```python
from build123d import *

# Parameters (mm, degrees)
BOSS_EXTRUDE1_DEPTH = 30
SKETCH2_R           = 7
SKETCH2_R_2         = 1.5
CUT_EXTRUDE1_DEPTH  = 55
SKETCH3_R           = 3
CUT_EXTRUDE2_DEPTH  = 55
SKETCH4_W           = 8
SKETCH4_H           = 40
BOSS_EXTRUDE2_DEPTH = 60
SKETCH5_R           = 2.5
CUT_EXTRUDE3_DEPTH  = 10
SKETCH6_W           = 8
SKETCH6_H           = 7.5
CUT_EXTRUDE4_DEPTH  = 94.808315196


with BuildPart() as part:
    # Sketch1 → Boss-Extrude1 (new, symmetric)
    with BuildSketch(Plane(origin=(0, 0, 0), x_dir=(0, 0, -1), z_dir=(1, 0, 0))):
        Polygon((0, 20), (0, 0), (-52, 0), (-52, -8), (8, -8), (8, 20), align=None)
    extrude(amount=BOSS_EXTRUDE1_DEPTH, both=True)

    # Sketch2 → Cut-Extrude1 (cut)
    with BuildSketch(Plane(origin=(0, 0, 0), x_dir=(1, 0, 0), z_dir=(0, 1, 0))):
        with Locations(Location((0, -37, 0), (0, 0, 270))):
            Circle(SKETCH2_R)
        with Locations(Location((15.75, -30, 0), (0, 0, 270))):
            Circle(SKETCH2_R_2)
        with Locations(Location((7.875, -43.63990011, 0), (0, 0, 270))):
            Circle(SKETCH2_R_2)
        with Locations(Location((-7.875, -43.63990011, 0), (0, 0, 270))):
            Circle(SKETCH2_R_2)
        with Locations(Location((-15.75, -30, 0), (0, 0, 270))):
            Circle(SKETCH2_R_2)
        with Locations(Location((-7.875, -16.36009989, 0), (0, 0, 270))):
            Circle(SKETCH2_R_2)
        with Locations(Location((7.875, -16.36009989, 0), (0, 0, 270))):
            Circle(SKETCH2_R_2)
    extrude(amount=-CUT_EXTRUDE1_DEPTH, mode=Mode.SUBTRACT)

    # Sketch3 → Cut-Extrude2 (cut)
    with BuildSketch(Plane.XY):
        with Locations((0, 12)):
            Circle(SKETCH3_R)
    extrude(amount=-CUT_EXTRUDE2_DEPTH, mode=Mode.SUBTRACT)

    # Sketch4 → Boss-Extrude2 (add)
    with BuildSketch(Plane(origin=(30, 0, 0), x_dir=(0, 0, -1), z_dir=(1, 0, 0))):
        with Locations((-56, -20)):
            Rectangle(SKETCH4_W, SKETCH4_H)
    extrude(amount=-BOSS_EXTRUDE2_DEPTH)

    # Sketch5 → Cut-Extrude3 (cut)
    with BuildSketch(Plane.XY.offset(60)):
        with Locations((25, -25.75)):
            Circle(SKETCH5_R)
        with Locations((-25, -25.75)):
            Circle(SKETCH5_R)
    extrude(amount=-CUT_EXTRUDE3_DEPTH, mode=Mode.SUBTRACT)

    # Sketch6 → Cut-Extrude4 (cut, through all)
    with BuildSketch(Plane.ZY.offset(30)):
        with Locations((56, -36.25)):
            Rectangle(SKETCH6_W, SKETCH6_H)
    extrude(amount=-CUT_EXTRUDE4_DEPTH, mode=Mode.SUBTRACT)


solid = part.part
```
Verification items for the finished model (mm, model axes). A direction names the side the tool comes from. Give positions to 0.01 mm unless a question says otherwise; leave off trailing zeros. Order: outer loops, then holes, each group sorted by start corner. A loop starts at its lowest first (then second) coordinate and runs counter-clockwise, first axis right, second up. Notation, with made-up numbers: M -12,46.25 L 14,46.25 A27 ccw 14,68.25 Z; hole C 79,21.25 d11. An arc over 180 degrees is marked long. Answer in a Markdown table with one row per item. Add a question column.
Item 1: Section check B-B, the plane y = -25.75. Enter the section's corners in (x, z).
Item 2: Section check C-C, the plane x = 26.5. Enter the section's corners in (y, z), and give its area (3 significant figures).
Item 3: Mould release check, pull along Z, two halves, no side actions. Record for faces 1 (the cylindrical face through (7.3, -3.944, 17.746)), 2 (the flat face through (0, -16, 60)), 3 (the cylindrical face through (-26.84, -24.06, 56.06)): released by +Z, released by -Z, zero draft, split by the parting line, or undercut.
Item 4: Scan lines: probe 1 along Y at (x, z) = (25, 57); probe 2 along X at (y, z) = (-6.5, 37); probe 3 along Y at (x, z) = (27, 10). Record each from-to range of solid material in increasing order. Write a range as from..to.
Item 5: Tool access check on faces 4 (the flat face through (0, 8, 0)), 5 (the flat face through (0, -8, 22)), 6 (the cylindrical face through (-8.45, -3.944, 17.746)). Record the directions out of +Z, -Z, +X, -X, +Y, -Y that give a thin tool (end or side, any length) a straight path to the whole face; none if there is none.
Item 6: Section check D-D, the plane y = 12. Enter the section's corners in (x, z), and give its area (3 significant figures).
Item 7: Gauge pin test, flat ends, axial feed: pin 1 (2.5 mm diameter, centred on x = -7.88, z = 43.64, fed in from -Y); pin 2 (4 mm diameter, centred on x = -7.88, z = 16.36, fed in from +Y); pin 3 (6.5 mm diameter, centred on x = -25, y = -25.75, fed in from -Z); pin 4 (5 mm diameter, centred on x = 15.75, z = 30, fed in from -Y). Record the tip position at first contact, or that the pin passes through.
Item 8: Section check A-A, the plane x = 0. Enter the section's corners in (y, z).
Filled sheet:
| question | item | result |
|---|---|---|
| 1 | outline | M -30,52 L -27.5,52 L -27.5,60 L -30,60 Z; M -22.5,52 L 22.5,52 L 22.5,60 L -22.5,60 Z; M 27.5,52 L 30,52 L 30,60 L 27.5,60 Z |
| 2 | outline | M -32.5,52 L -27.75,52 L -27.75,60 L -32.5,60 Z; M -23.75,52 L -8,52 L -8,-8 L 20,-8 L 20,0 L 0,0 L 0,60 L -23.75,60 Z |
| 2 | area | 868 mm^2 |
| 3 | face 1 | undercut |
| 3 | face 2 | released by +Z |
| 3 | face 3 | zero draft |
| 4 | probe 1 | y = -32.5..-28.25, -23.25..0 |
| 4 | probe 2 | x = -30..-7, 7..30 |
| 4 | probe 3 | y = -8..0 |
| 5 | face 4 | +Z, +X, -X, +Y |
| 5 | face 5 | -Z, +X, -X, -Y |
| 5 | face 6 | +Y, -Y |
| 6 | outline | M -30,-8 L -3,-8 L -3,0 L -30,0 Z; M 3,-8 L 30,-8 L 30,0 L 3,0 Z |
| 6 | area | 432 mm^2 |
| 7 | pin 1 | passes through |
| 7 | pin 2 | stops at y = 0 |
| 7 | pin 3 | stops at z = 52 |
| 7 | pin 4 | stops at y = -8 |
| 8 | outline | M -32.5,52 L -8,52 L -8,44 L 0,44 L 0,60 L -32.5,60 Z; M -8,-8 L 9,-8 L 9,0 L 0,0 L 0,30 L -8,30 Z; M 15,-8 L 20,-8 L 20,0 L 15,0 Z |
